```python
from build123d import *

# Parameters (mm, degrees)
ESBO_O1_R                = 2
RESSALTO_EXTRUS_O1_DEPTH = 7
ESBO_O2_R                = 3.5
RESSALTO_EXTRUS_O2_DEPTH = 12
ESBO_O3_R                = 1.975
CORTE_EXTRUS_O1_DEPTH    = 8


with BuildPart() as part:
    # Esboço1 → Ressalto-extrusão1 (new body)
    with BuildSketch(Plane.XY):
        Polygon((0, 4.613028651), (-3.995, 2.306514325), (-3.995, -2.306514325), (0, -4.613028651), (3.995, -2.306514325), (3.995, 2.306514325), align=None)
        Circle(ESBO_O1_R, mode=Mode.SUBTRACT)
    extrude(amount=RESSALTO_EXTRUS_O1_DEPTH)

    # Esboço2 → Ressalto-extrusão2 (add)
    with BuildSketch(Plane.XY.offset(7)):
        Circle(ESBO_O2_R)
    extrude(amount=RESSALTO_EXTRUS_O2_DEPTH)

    # Esboço3 → Corte-extrusão1 (cut)
    with BuildSketch(Plane.XY.offset(19)):
        Circle(ESBO_O3_R)
    extrude(amount=-CORTE_EXTRUS_O1_DEPTH, mode=Mode.SUBTRACT)


solid = part.part
```
Geometry check sheet. Reference: the model listing, model coordinates, mm. A direction names the side the tool comes from. Coordinates: 2 decimals unless noted, no trailing zeros. Order: outer loops, then holes, each group sorted by start corner. A loop starts at its lowest first (then second) coordinate and runs counter-clockwise, first axis right, second up. Notation, with made-up numbers: (62.5, 55) - (81.5, 55) arc R27 cw to (81.5, 75) - close; hole circle Ø2 at (72.25, -8). An arc over 180 degrees is marked (long way). Answer as a JSON object with one key per item and string values. Group by question number.
Item 1: Scan lines: probe 1 along Y at (x, z) = (0, 17) (3 decimals); probe 2 along Y at (x, z) = (1.5, 15.5); probe 3 along X at (y, z) = (-0.75, 3.75) (3 decimals). Record each from-to range of solid material in increasing order.
Item 2: Draft check along X on faces 1 (the face through (2.03, 3.44, 3.45)), 2 (the face through (-2, -1, 0)), 3 (the face through (-1.57, -1.2, 15.06)). Enter one of: +X half, -X half, draft (parallel to the pull), parting line (faces both ways), or undercut.
Item 3: Tool access check on faces 4 (the face through (0, 0, 11)), 5 (the face through (-1.97, 3.476, 3.451)), 6 (the face through (0, 0, 7)). Record the directions out of +Z, -Z, +X, -X, +Y, -Y that give a thin tool (end or side, any length) a straight path to the whole face; none if there is none.
Item 4: Sectioned sample at C-C, the plane x = -1.25. Record the cut outline in (y, z), and give its area (3 significant figures).
Item 5: Depth check by flat-ended pin: pin 1 Ø1 at (x, z) = (1, 15.5) entering from -Y; pin 2 Ø1.2 at (x, y) = (0, 0) entering from -Z; pin 3 Ø3.5 at (x, y) = (0, 0) entering from +Z. Enter the tip coordinate at first touch or a pass-through.
Item 6: Sectioned sample at B-B, the plane z = 4. Record the cut outline in (x, y) (3 decimals), and give its area (3 significant figures).
Item 7: Sectioned sample at D-D, the plane z = 10.75. Record the cut outline in (x, y), and give its area (3 significant figures).
Item 8: Sectioned sample at A-A, the plane y = 0. Record the cut outline in (x, z) (3 decimals).
Resolved:
{
 "1": {"probe 1": "-3.5 to -1.975, 1.975 to 3.5", "probe 2": "-3.16 to -1.28, 1.28 to 3.16", "probe 3": "-3.995 to -1.854, 1.854 to 3.995"},
 "2": {"face 1": "+X half", "face 2": "draft", "face 3": "undercut"},
 "3": {"face 4": "+Z", "face 5": "+Z, -Z, -X, +Y", "face 6": "-Z"},
 "4": {"outline": "(-3.89, 0) - (-1.56, 0) - (-1.56, 7) - (1.56, 7) - (1.56, 0) - (3.89, 0) - (3.89, 7) - (3.27, 7) - (3.27, 19) - (1.53, 19) - (1.53, 11) - (-1.53, 11) - (-1.53, 19) - (-3.27, 19) - (-3.27, 7) - (-3.89, 7) - close", "area": "86.6 mm^2"},
 "5": {"pin 1": "y = -3.46", "pin 2": "z = 7", "pin 3": "z = 11"},
 "6": {"outline": "(-3.995, -2.307) - (0, -4.613) - (3.995, -2.307) - (3.995, 2.307) - (0, 4.613) - (-3.995, 2.307) - close; hole circle Ø4 at (0, 0)", "area": "42.7 mm^2"},
 "7": {"outline": "circle Ø7 at (0, 0)", "area": "38.5 mm^2"},
 "8": {"outline": "(-3.995, 0) - (-2, 0) - (-2, 7) - (2, 7) - (2, 0) - (3.995, 0) - (3.995, 7) - (3.5, 7) - (3.5, 19) - (1.975, 19) - (1.975, 11) - (-1.975, 11) - (-1.975, 19) - (-3.5, 19) - (-3.5, 7) - (-3.995, 7) - close"}
}
